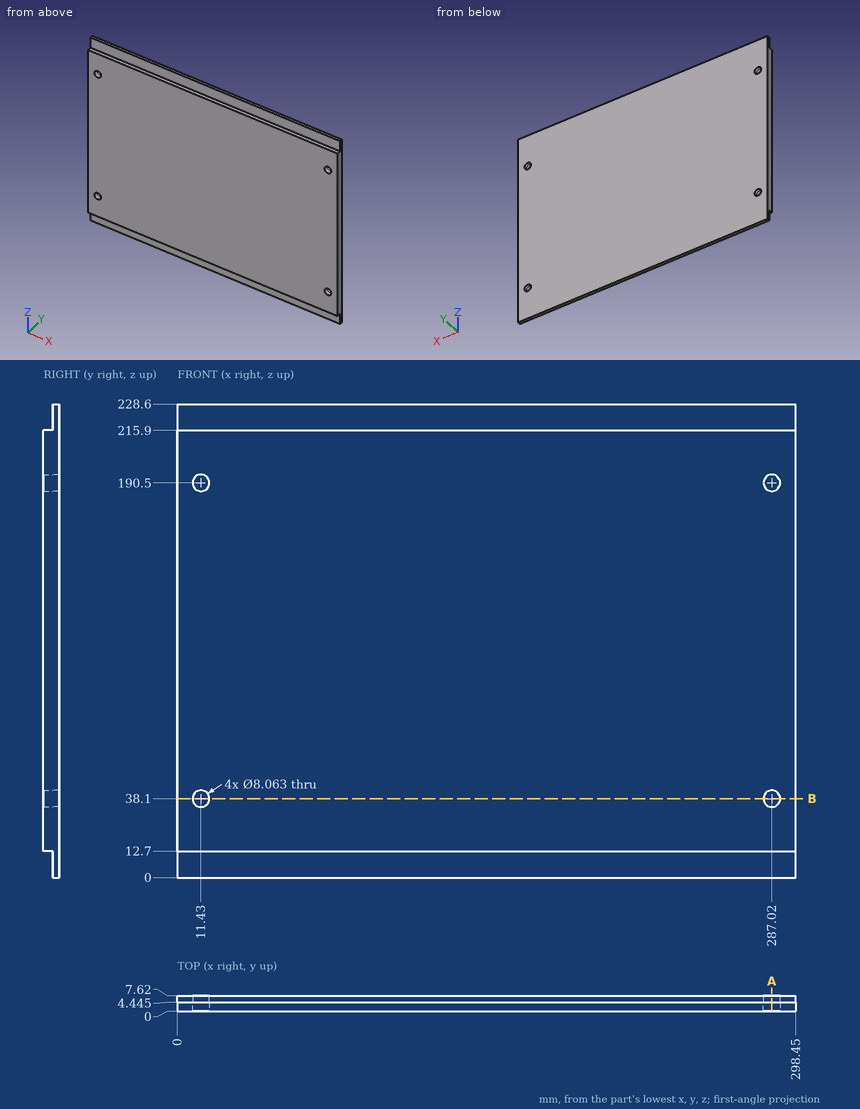
Geometry check sheet. Reference: drawing and pictorial views, mm from the part's lowest x, y, z. Coordinates: 2 decimals unless noted, no trailing zeros. Loops run counter-clockwise (first coordinate to the right, second up) from the corner with the lowest first, then second, coordinate; pieces in that order, holes last.
1) Sectioned sample at B-B (z = 38.1). Record the boundary of the cut face in (x, y).
2) Sectioned sample at A-A (x = 287.02). Record the boundary of the cut face in (y, z) (1 decimal), and give its area (3 significant figures).
3) Gauge pin test, flat ends, axial feed: pin 1 (3.5 mm diameter, centred on x = 215, y = 2.5, fed in from -Z); pin 2 (6.5 mm diameter, centred on x = 145, z = 220.5, fed in from -Y) (3 decimals); pin 3 (3.5 mm diameter, centred on x = 204.5, y = 2, fed in from +Z). Record the tip position at first contact, or that the pin passes through.
4) Material ranges on probe 1 along Z at (x, y) = (11.43, 6.6); probe 2 along Z at (x, y) = (11.43, 1.4); probe 3 along X at (y, z) = (2.65, 190.5), recorded low to high.
Check sheet entries:
1. outline: (0, 0) - (7.4, 0) - (7.4, 7.62) - (0, 7.62) - close; (15.46, 0) - (282.99, 0) - (282.99, 7.62) - (15.46, 7.62) - close; (291.05, 0) - (298.45, 0) - (298.45, 7.62) - (291.05, 7.62) - close
2. outline: (0, 12.7) - (4.4, 12.7) - (4.4, 0) - (7.6, 0) - (7.6, 34.1) - (0, 34.1) - close; (0, 42.1) - (7.6, 42.1) - (7.6, 186.5) - (0, 186.5) - close; (0, 194.5) - (7.6, 194.5) - (7.6, 228.6) - (4.4, 228.6) - (4.4, 215.9) - (0, 215.9) - close
2. area: 1,510 mm2
3. pin 1: stops at z = 12.7
3. pin 2: stops at y = 4.445
3. pin 3: stops at z = 215.9
4. probe 1: z = 0 to 34.07, 42.13 to 186.47, 194.53 to 228.6
4. probe 2: z = 12.7 to 34.07, 42.13 to 186.47, 194.53 to 215.9
4. probe 3: x = 0 to 7.4, 15.46 to 282.99, 291.05 to 298.45
